from build123d import *

# Parameters (mm, degrees)
SKETCH1_W             = 50
SKETCH1_H             = 55
BOSS_EXTRUDE1_DEPTH   = 40
SKETCH2_R             = 14
CUT_EXTRUDE1_DEPTH    = 55.60082417
M5_TAPPED_HOLE1_D     = 4.2
M5_TAPPED_HOLE1_DEPTH = 15
M5_TAPPED_HOLE1_TIP   = 1.2618073
M5_TAPPED_HOLE3_D     = 4.2
M5_TAPPED_HOLE3_DEPTH = 17.4
M5_TAPPED_HOLE3_TIP   = 1.2618073


with BuildPart() as part:
    # Sketch1 → Boss-Extrude1 (new body)
    with BuildSketch(Plane.XY):
        Rectangle(SKETCH1_W, SKETCH1_H)
    extrude(amount=-BOSS_EXTRUDE1_DEPTH)

    # Sketch2 → Cut-Extrude1 (cut, through all)
    with BuildSketch(Plane.XY):
        with Locations((0, 4.5)):
            Circle(SKETCH2_R)
    extrude(amount=-CUT_EXTRUDE1_DEPTH, mode=Mode.SUBTRACT)

    # M5 Tapped Hole1
    with Locations(Plane(origin=(-20, -27.5, -8), x_dir=(-1, 0, 0), z_dir=(0, -1, 0))):
        with Locations((0, 0), (-40, 0), (-40, 24), (0, 24)):
            Hole(M5_TAPPED_HOLE1_D / 2, depth=M5_TAPPED_HOLE1_DEPTH)
            with Locations((0, 0, -(M5_TAPPED_HOLE1_DEPTH + M5_TAPPED_HOLE1_TIP / 2))):  # 118° drill point
                Cone(0, M5_TAPPED_HOLE1_D / 2, M5_TAPPED_HOLE1_TIP, mode=Mode.SUBTRACT)

    # M5 Tapped Hole3
    with Locations(Plane(origin=(13.435028843, 17.935028843, 0), x_dir=(1, 0, 0), z_dir=(0, 0, 1))):
        with Locations((0, 0), (0, -26.870057686), (-26.870057686, -26.870057686), (-26.870057686, 0)):
            Hole(M5_TAPPED_HOLE3_D / 2, depth=M5_TAPPED_HOLE3_DEPTH)
            with Locations((0, 0, -(M5_TAPPED_HOLE3_DEPTH + M5_TAPPED_HOLE3_TIP / 2))):  # 118° drill point
                Cone(0, M5_TAPPED_HOLE3_D / 2, M5_TAPPED_HOLE3_TIP, mode=Mode.SUBTRACT)


solid = part.part
The listing builds one solid part. Answer for the finished solid, in the listing's coordinates (mm). A direction names the side the tool comes from. Round coordinates to 2 decimals unless told otherwise and drop trailing zeros. Write each loop counter-clockwise with the first axis right and the second up, starting at its lowest first coordinate (ties: lowest second). Pieces come first, ordered by that corner, then holes. Notation, with made-up numbers: M 25,87.5 L 79,87.5 A27 cw 79,107.5 Z; hole C 32.25,14.25 d5. An arc over 180 degrees is marked long. Write each question's results on one line, items separated by ' | '. Start each with the question number.
Item 1: Find section C-C on z = -11.5. Write down the section's boundary in (x, y), and give its area (3 significant figures).
Item 2: Find section B-B on x = -1.5. Write down the section's boundary in (y, z).
Item 3: Find section A-A on y = 4.5. Write down the section's boundary in (x, z).
Item 4: Straight lines are drawn through the part: probe 1 along X at (y, z) = (-18, -32); probe 2 along X at (y, z) = (5, -23); probe 3 along Z at (x, y) = (-19.5, -12.5). For each, find the intervals that lie inside material, in ascending order.
Item 5: The mould has two halves that part along Y. Classify faces 1 (the cylindrical face through (13.708, -6.853, -8.822)), 2 (the conical face through (20.364, -11.457, -32.016)), 3 (the flat face through (-25, 0, -20)), 4 (the flat face through (0, 27.5, -20)): +Y half, -Y half, draft (parallel to the pull), parting line (faces both ways), or undercut.
Item 6: Find section D-D on y = -17. Write down the section's boundary in (x, z), and give its area (3 significant figures).
Item 7: Given pin 1 Ø5 at (x, y) = (-1, -5.5) entering from -Z; pin 2 Ø3.5 at (x, y) = (13.44, 17.94) entering from +Z; pin 3 Ø3.5 at (x, z) = (-20, -8) entering from -Y, each flat-ended and moving along its own axis, determine where each tip first touches the part or whether it passes through.
Item 8: Which of the six approach directions +Z, -Z, +X, -X, +Y, -Y give full straight-line access (tool end or side, diameter ignored) to faces 5 (the cylindrical face through (20.969, -19.895, -30.137)), 6 (the cylindrical face through (13.35, 8.71, -19.72)), 7 (the cylindrical face through (13.89, 15.885, -8.822))?
Answer block:
1) outline: M -25,-27.5 L 25,-27.5 L 25,27.5 L -25,27.5 Z; hole C -13.44,-8.94 d4.2; hole C -13.44,17.94 d4.2; hole C 0,4.5 d28; hole C 13.44,-8.94 d4.2; hole C 13.44,17.94 d4.2 | area: 2,080 mm²
2) outline: M -27.5,-40 L -9.42,-40 L -9.42,0 L -27.5,0 Z; M 18.42,-40 L 27.5,-40 L 27.5,0 L 18.42,0 Z
3) outline: M -25,-40 L -14,-40 L -14,0 L -25,0 Z; M 14,-40 L 25,-40 L 25,0 L 14,0 Z
4) probe 1: x = -25 to -22.1, -17.9 to 17.9, 22.1 to 25 | probe 2: x = -25 to -13.99, 13.99 to 25 | probe 3: z = -40 to -34.04, -29.96 to -10.04, -5.96 to 0
5) face 1: undercut | face 2: -Y half | face 3: draft | face 4: +Y half
6) outline: M -25,-40 L 25,-40 L 25,0 L -25,0 Z; hole C -20,-32 d4.2; hole C -20,-8 d4.2; hole C 20,-32 d4.2; hole C 20,-8 d4.2 | area: 1,940 mm²
7) pin 1: passes through | pin 2: stops at z = -17.61 | pin 3: stops at y = -12.29
8) face 5: -Y | face 6: +Z, -Z | face 7: +Z
